Autodesk Inventor part; units mm, degrees
ref_plane "YZ Plane" through (0, 0, 0) normal (1, 0, 0) x (0, 1, 0)
ref_plane "XZ Plane" through (0, 0, 0) normal (0, 1, 0) x (-1, 0, 0)
ref_plane "XY Plane" through (0, 0, 0) normal (0, 0, 1) x (1, 0, 0)
sketch "Эскиз1" plane through (0, 0, 0) normal (0, 0, 1) x (1, 0, 0)
  line L0 (74.0863, 52.032) -> (-90.9137, 52.032)
  line L1 (-90.9137, 52.032) -> (-90.9137, 5.032)
  line L2 (-90.9137, 5.032) -> (74.0863, 5.032)
  line L3 (74.0863, 5.032) -> (74.0863, 52.032)
  point P0 (0, 0)
  dimension "d0" = 47
  dimension "d1" = 165
extrude "Выдавливание1" add sketch "Эскиз1" along normal blind 38
fillet "Сопряжение1" radius 15 2 edges at (74.0863, 28.532, 38) (74.0863, 28.532, 0)
properties part number "akkum16v"
Source: CAD feature listing. Evaluate the final solid. Frame: model axes, mm. Coordinates: 2 decimals unless noted, no trailing zeros. Loops run counter-clockwise (first coordinate to the right, second up) from the corner with the lowest first, then second, coordinate; pieces in that order, holes last. Notation, with made-up numbers: (66, 51) -> (101, 51) arc R16 cw to (101, 78) -> close; hole circle Ø7 at (-26, -32). An arc over 180 degrees is marked (long way). One line per item, written item: value. Start each with the question number.
Q1. Contact query for flat-ended pins moving along their axis: P1, Ø10, axis at x = -61, y = 39, coming from the -Z side; P2, Ø2, axis at y = 41, z = 13, coming from the +X side. Output: stop coordinate, or through.
Q2. Line query: line 1 along X through (y, z) = (15.5, 36); line 2 along X through (y, z) = (26, 31.5); line 3 along Z through (x, y) = (67, 8.5). Output: solid intervals per line, ascending.
Q3. Section query B-B, the plane z = 6. Return the cut outline in (x, y).
Q4. Section query A-A, the plane y = 27.5. Return the cut outline in (x, z).
Results:
1. P1: z = 0
1. P2: x = 74.05
2. line 1: -90.91 to 66.57
2. line 2: -90.91 to 71.45
2. line 3: 2.26 to 35.74
3. outline: (-90.91, 5.03) -> (71.09, 5.03) -> (71.09, 52.03) -> (-90.91, 52.03) -> close
4. outline: (-90.91, 0) -> (59.09, 0) arc R15 ccw to (74.09, 15) -> (74.09, 23) arc R15 ccw to (59.09, 38) -> (-90.91, 38) -> close
